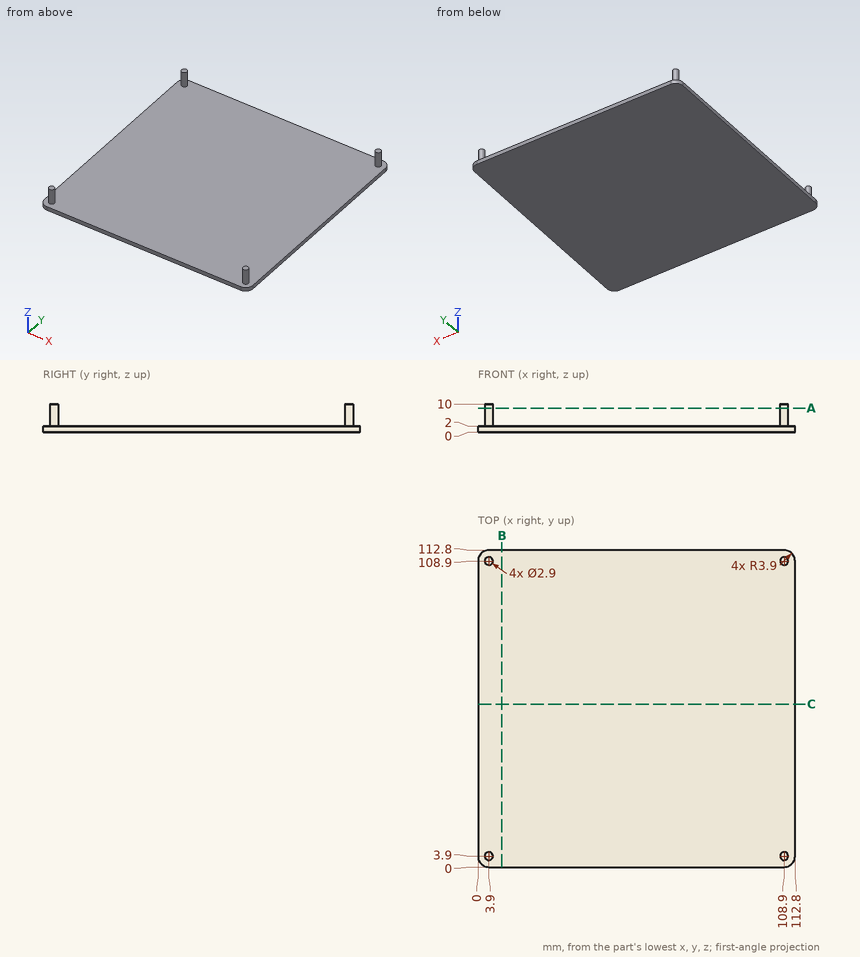
Geometry check sheet. Reference: drawing and pictorial views, mm from the part's lowest x, y, z. Round coordinates to 2 decimals unless told otherwise and drop trailing zeros. Write each loop counter-clockwise with the first axis right and the second up, starting at its lowest first coordinate (ties: lowest second). Pieces come first, ordered by that corner, then holes.
1. Section check B-B on x = 8.5. Enter the section's corners in (y, z), plus the area to 3 significant figures.
2. Gauge pin test, flat ends, axial feed: P1, Ø1, axis at x = 11.5, y = 27, coming from the -Z side; P2, Ø3, axis at y = 90, z = 4, coming from the +X side. Record the tip position at first contact, or that the pin passes through.
3. Section check A-A on z = 8.5. Enter the section's corners in (x, y).
4. Scan lines: L1, parallel to Z at x = 64.5, y = 72.5; L2, parallel to Y at x = 5, z = 5.25. Record each from-to range of solid material in increasing order.
Answer:
1. outline: (0, 0) - (112.8, 0) - (112.8, 2) - (0, 2) - close
1. area: 226 mm2
2. P1: stops at z = 0
2. P2: passes through
3. outline: circle Ø2.9 at (3.9, 3.9); circle Ø2.9 at (3.9, 108.9); circle Ø2.9 at (108.9, 3.9); circle Ø2.9 at (108.9, 108.9)
4. L1: z = 0 to 2
4. L2: y = 2.96 to 4.84, 107.96 to 109.84
